```python
from build123d import *

# Parameters (mm, degrees)
ESQUISSE1_W             = 300
ESQUISSE1_H             = 52
BOSS_EXTRU_1_DEPTH      = 8
ESQUISSE2_W             = 8
ESQUISSE2_H             = 10
ENL_V_MAT_EXTRU_1_DEPTH = 153.446712001
ESQUISSE3_W             = 8
ESQUISSE3_H             = 2
ENL_V_MAT_EXTRU_2_DEPTH = 153.446712001
ENL_V_MAT_EXTRU_3_DEPTH = 153.446712001
ESQUISSE5_W             = 15
ESQUISSE5_H             = 8
ENL_V_MAT_EXTRU_4_DEPTH = 10


with BuildPart() as part:
    # Esquisse1 → Boss.-Extru.1 (new body)
    with BuildSketch(Plane.XY):
        Rectangle(ESQUISSE1_W, ESQUISSE1_H)
    extrude(amount=BOSS_EXTRU_1_DEPTH)

    # Esquisse2 → Enlèv. mat.-Extru.1 (cut, through all)
    with BuildSketch(Plane.XY):
        with Locations((-146, 1)):
            Rectangle(ESQUISSE2_W, ESQUISSE2_H)
        with Locations((-146, 21)):
            Rectangle(ESQUISSE2_W, ESQUISSE2_H)
        with Locations((-146, -19)):
            Rectangle(ESQUISSE2_W, ESQUISSE2_H)
    enl_v_mat_extru_1 = extrude(amount=ENL_V_MAT_EXTRU_1_DEPTH, mode=Mode.SUBTRACT)

    # Esquisse3 → Enlèv. mat.-Extru.2 (cut, through all)
    with BuildSketch(Plane.XY):
        with Locations((-146, -25)):
            Rectangle(ESQUISSE3_W, ESQUISSE3_H)
    enl_v_mat_extru_2 = extrude(amount=ENL_V_MAT_EXTRU_2_DEPTH, mode=Mode.SUBTRACT)

    # Symétrie1: Enlèv. mat.-Extru.1, Enlèv. mat.-Extru.2 across plane
    add(enl_v_mat_extru_1.mirror(Plane(origin=(0, 0, 0), x_dir=(0, 0, 1), z_dir=(1, 0, 0))), mode=Mode.SUBTRACT)
    add(enl_v_mat_extru_2.mirror(Plane(origin=(0, 0, 0), x_dir=(0, 0, 1), z_dir=(1, 0, 0))), mode=Mode.SUBTRACT)

    # Esquisse4 → Enlèv. mat.-Extru.3 (cut, through all)
    with BuildSketch(Plane.XY):
        with BuildLine():
            Line((-100, 12.5), (100, 12.5))
            ThreePointArc((100, 12.5), (112.5, 0), (100, -12.5))
            Line((100, -12.5), (-100, -12.5))
            ThreePointArc((-100, -12.5), (-112.5, 0), (-100, 12.5))
        make_face()
    extrude(amount=ENL_V_MAT_EXTRU_3_DEPTH, mode=Mode.SUBTRACT)

    # Esquisse5 → Enlèv. mat.-Extru.4 (cut)
    with BuildSketch(Plane.XY):
        Polygon((0, 26), (-15, 26), (-15, 18), (0, 18), (14.777360912, 18), (14.777360912, 26), align=None)
        with Locations((-37.5, 22)):
            Rectangle(ESQUISSE5_W, ESQUISSE5_H)
        with Locations((-67.5, 22)):
            Rectangle(ESQUISSE5_W, ESQUISSE5_H)
        with Locations((-97.5, 22)):
            Rectangle(ESQUISSE5_W, ESQUISSE5_H)
        with Locations((37.5, 22)):
            Rectangle(ESQUISSE5_W, ESQUISSE5_H)
        with Locations((67.5, 22)):
            Rectangle(ESQUISSE5_W, ESQUISSE5_H)
        with Locations((97.5, 22)):
            Rectangle(ESQUISSE5_W, ESQUISSE5_H)
    extrude(amount=ENL_V_MAT_EXTRU_4_DEPTH, mode=Mode.SUBTRACT)


solid = part.part
```
Build history of the part. All positions in model axes, mm. A direction names the side the tool comes from. Give positions to 0.01 mm unless a question says otherwise; leave off trailing zeros. Loops run counter-clockwise (first coordinate to the right, second up) from the corner with the lowest first, then second, coordinate; pieces in that order, holes last. Notation, with made-up numbers: (54.5, 42) -> (77.5, 42) arc R34 cw to (77.5, 76) -> close; hole circle Ø4 at (38.5, 53). An arc over 180 degrees is marked (long way). One line per question, with ' | ' between items.
Q1. Cut at A-A, the plane y = 0. Write the cut outline in (x, z).
Filled sheet:
outline: (-142, 0) -> (-112.5, 0) -> (-112.5, 8) -> (-142, 8) -> close; (112.5, 0) -> (142, 0) -> (142, 8) -> (112.5, 8) -> close
Q2. Pull direction Y, two halves, no side cores. Call faces 1 (the flat face through (-146, -14, 4)), 2 (the flat face through (-90, 22, 4)), 3 (the cylindrical face through (-112.497, -0.275, 3.944)): pulls with the +Y half, pulls with the -Y half, needs draft (parallel to the pull), parting line crosses it, or undercut.
Filled sheet:
face 1: pulls with the -Y half | face 2: needs draft | face 3: undercut
Q3. Tool access for faces 4 (the flat face through (-15, 22, 4)), 5 (the flat face through (-146, 6, 4)), 6 (the flat face through (-142, 21, 4)), 7 (the flat face through (142, 21, 4)): list every direction of +Z, -Z, +X, -X, +Y, -Y with a clear straight run to the whole face (end or side of a thin tool).
Filled sheet:
face 4: +Z, -Z, +Y | face 5: +Z, -Z, -X | face 6: +Z, -Z, -X, +Y | face 7: +Z, -Z, +X, +Y
Q4. Drill centre lines: line 1 along Y through (x, z) = (74.5, 0.5); line 2 along Y through (x, z) = (-51, 2); line 3 along X through (y, z) = (-10, 3.25). Where is each one in solid material? Low to high. Write a range as [from, to].
Filled sheet:
line 1: y = [-26, -12.5], [12.5, 18] | line 2: y = [-26, -12.5], [12.5, 26] | line 3: x = [-150, -107.5], [107.5, 150]
Q5. Drop flat-ended pins along their axis: pin 1 (1.5 mm diameter, centred on y = -1.5, z = 4.5, fed in from -X); pin 2 (4 mm diameter, centred on y = 23.5, z = 3.5, fed in from +X). Give the stop position or say it passes through.
Filled sheet:
pin 1: stops at x = -142 | pin 2: stops at x = 142
Q6. Cut at B-B, the plane x = 41. Write the cut outline in (y, z).
Filled sheet:
outline: (-26, 0) -> (-12.5, 0) -> (-12.5, 8) -> (-26, 8) -> close; (12.5, 0) -> (18, 0) -> (18, 8) -> (12.5, 8) -> close
